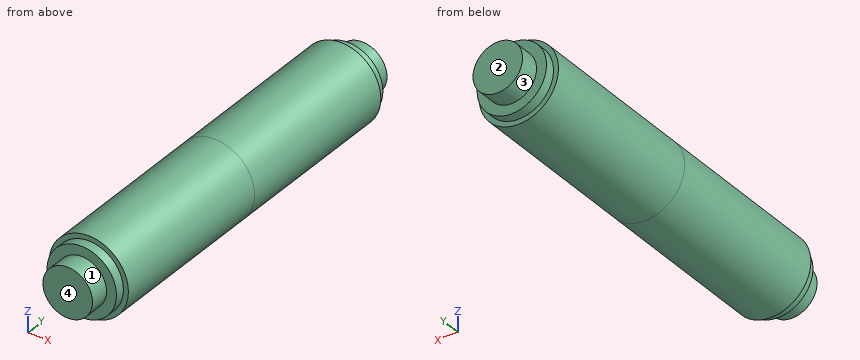
from build123d import *


with BuildPart() as part:
    # Sketch1 → Revolve1 (revolve)
    with BuildSketch(Plane.XY):
        Polygon((0, 21), (0, 0), (4, 0), (4, 18), (3.5, 18), (3.5, 19), (2.5, 19), (2.5, 21), align=None)
    revolve1 = revolve(axis=Axis((0, 21, 0), (0, -1, 0)))

    # Mirror1: Revolve1 across plane
    add(revolve1.mirror(Plane.ZX))


solid = part.part
Check sheet for the modelled part. Datum: model origin and axes. Units: mm. Face numbers are marked on the shaded views. A direction names the side the tool comes from. Give positions to 0.01 mm unless a question says otherwise; leave off trailing zeros. Loops run counter-clockwise (first coordinate to the right, second up) from the corner with the lowest first, then second, coordinate; pieces in that order, holes last. Notation, with made-up numbers: M 57.5,16 L 80.5,16 A25 cw 80.5,55 Z; hole C 42.25,57.5 d7. An arc over 180 degrees is marked long. Return JSON: item names as keys, results as strings. Group by question number.
1. Cross-section at D-D on x = -3. Record the boundary of the cut face in (y, z).
2. Thickness scan on L1, parallel to Y at x = 2.5, z = -1.5; L2, parallel to Y at x = -2.25, z = -3.25; L3, parallel to X at y = 5.5, z = -2. Record the ranges inside material, lowest first.
3. Cross-section at C-C on y = -4. Record the boundary of the cut face in (x, z).
4. Cross-section at B-B on z = 0. Record the boundary of the cut face in (x, y), plus the area to 3 significant figures.
5. Go/stop test with a flat-tipped pin: pin 1 (2 mm diameter, centred on x = -2.5, z = 1, fed in from -Y). Record where the tip stops, or that it passes through.
6. Cross-section at A-A on x = 0. Record the boundary of the cut face in (y, z), plus the area to 3 significant figures.
7. Tool access check on the marked faces 1 and 2. Record the directions out of +Z, -Z, +X, -X, +Y, -Y that give a thin tool (end or side, any length) a straight path to the whole face; none if there is none.
8. Mould release check, pull along X, two halves, no side actions. Record for the marked faces 3 and 4: released by +X, released by -X, zero draft, split by the parting line, or undercut.
Return value:
{
 "1": {"outline": "M -19,-1.8 L -18,-1.8 L -18,-2.65 L 18,-2.65 L 18,-1.8 L 19,-1.8 L 19,1.8 L 18,1.8 L 18,2.65 L -18,2.65 L -18,1.8 L -19,1.8 Z"},
 "2": {"L1": "-19 to 19", "L2": "-18 to 18", "L3": "-3.46 to 3.46"},
 "3": {"outline": "C 0,0 d8"},
 "4": {"outline": "M -4,-18 L -3.5,-18 L -3.5,-19 L -2.5,-19 L -2.5,-21 L 2.5,-21 L 2.5,-19 L 3.5,-19 L 3.5,-18 L 4,-18 L 4,18 L 3.5,18 L 3.5,19 L 2.5,19 L 2.5,21 L -2.5,21 L -2.5,19 L -3.5,19 L -3.5,18 L -4,18 Z", "area": "322 mm^2"},
 "5": {"pin 1": "y = -21"},
 "6": {"outline": "M -21,-2.5 L -19,-2.5 L -19,-3.5 L -18,-3.5 L -18,-4 L 18,-4 L 18,-3.5 L 19,-3.5 L 19,-2.5 L 21,-2.5 L 21,2.5 L 19,2.5 L 19,3.5 L 18,3.5 L 18,4 L -18,4 L -18,3.5 L -19,3.5 L -19,2.5 L -21,2.5 Z", "area": "322 mm^2"},
 "7": {"face 1": "-Y", "face 2": "+Z, -Z, +X, -X, +Y"},
 "8": {"face 3": "split by the parting line", "face 4": "zero draft"}
}
